Source: CAD feature listing. Evaluate the final solid. Frame: model axes, mm. A direction names the side the tool comes from. Give positions to 0.01 mm unless a question says otherwise; leave off trailing zeros. Loops run counter-clockwise (first coordinate to the right, second up) from the corner with the lowest first, then second, coordinate; pieces in that order, holes last. Notation, with made-up numbers: M 79.5,64.25 L 131.5,64.25 A18 ccw 131.5,71.25 Z; hole C 15,36 d7. An arc over 180 degrees is marked long. Put each result on its own line as item: value.
from build123d import *

# Parameters (mm, degrees)
SKETCH_1_W          = 50
SKETCH_1_H          = 20
EXTRUDE_1_DEPTH     = 180
CUT_EXTRUDE_1_DEPTH = 10
CUT_EXTRUDE_2_DEPTH = 10
SKETCH_4_OUTSIDE_W  = 219.576
SKETCH_4_OUTSIDE_H  = 89.576
CUT_EXTRUDE_4_DEPTH = 21


with BuildPart() as part:
    # Эскиз1 → Бобышка-Вытянуть1 (new body)
    with BuildSketch(Plane(origin=(0, 0, 0), x_dir=(0, 0, -1), z_dir=(1, 0, 0))):
        with Locations((25, 10)):
            Rectangle(SKETCH_1_W, SKETCH_1_H)
    extrude(amount=EXTRUDE_1_DEPTH)

    # Эскиз2 → Вырез-Вытянуть1 (cut)
    with BuildSketch(Plane.XZ):
        with BuildLine():
            Line((43.517527849, -50), (0, -50))
            Line((0, -50), (0, 0))
            Line((0, 0), (50.69898236, 0))
            Line((50.69898236, 0), (60.088568146, -16.308535178))
            ThreePointArc((60.088568146, -16.308535178), (60.755434633, -18.806330829), (60.085562557, -21.303322104))
            Line((60.085562557, -21.303322104), (43.517527849, -50))
        make_face()
    extrude(amount=-CUT_EXTRUDE_1_DEPTH, mode=Mode.SUBTRACT)

    # Эскиз3 → Вырез-Вытянуть2 (cut)
    with BuildSketch(Plane(origin=(0, 20, 0), x_dir=(1, 0, 0), z_dir=(0, 1, 0))):
        with BuildLine():
            Line((119.870060572, 21.260602823), (136.462759268, 50))
            Line((136.462759268, 50), (180, 50))
            Line((180, 50), (180, 0))
            Line((180, 0), (129.384239064, 0))
            Line((129.384239064, 0), (119.884637949, 16.23552237))
            ThreePointArc((119.884637949, 16.23552237), (119.200208629, 18.746098263), (119.870060572, 21.260602823))
        make_face()
    extrude(amount=-CUT_EXTRUDE_2_DEPTH, mode=Mode.SUBTRACT)

    # Эскиз4 outside → Вырез-Вытянуть4 (cut, through all)
    with BuildSketch(Plane(origin=(0, 20, 0), x_dir=(1, 0, 0), z_dir=(0, 1, 0))):
        with Locations((90, 25)):
            Rectangle(SKETCH_4_OUTSIDE_W, SKETCH_4_OUTSIDE_H)
        with BuildLine():
            Line((180, 50), (152.575862213, 2.5))
            ThreePointArc((152.575862213, 2.5), (150.745735195, 0.669872981), (148.245735195, 0))
            Line((148.245735195, 0), (31.754264805, 0))
            ThreePointArc((31.754264805, 0), (29.254264805, 0.669872981), (27.424137787, 2.5))
            Line((27.424137787, 2.5), (0, 50))
            Line((0, 50), (180, 50))
        make_face(mode=Mode.SUBTRACT)
    extrude(amount=-CUT_EXTRUDE_4_DEPTH, mode=Mode.SUBTRACT)


solid = part.part
1. Contact query for flat-ended pins moving along their axis: P1, Ø1.5, axis at y = 17.5, z = -12.5, coming from the +X side; P2, Ø5, axis at x = 147, z = -34, coming from the +Y side; P3, Ø10, axis at y = 10.5, z = -21.5, coming from the -X side. Output: stop coordinate, or through.
Found:
P1: x = 122.51
P2: y = 10
P3: x = 13.57
2. Draft query along Z for faces 1 (the flat face through (89, 10, -50)), 2 (the flat face through (111, 0, -25)), 3 (the cylindrical face through (119.2, 15.1, -18.7)), 4 (the flat face through (89, 10, 0)). Return one class per face: pulls with the +Z half, pulls with the -Z half, needs draft (parallel to the pull), parting line crosses it, or undercut.
Found:
face 1: pulls with the -Z half
face 2: needs draft
face 3: undercut
face 4: pulls with the +Z half
3. Material intervals for line 1 (Y direction, x = 29.5, z = -24.5); line 2 (Y direction, x = 150.5, z = -40.5); line 3 (X direction, y = 3, z = -12), sorted ascending. Write a range as from..to.
Found:
line 1: 10..20
line 2: 0..10
line 3: 57.61..158.06
4. Section query C-C (y = 4). Output: boundary loops of the cut face in (x, z), plus the area to 3 significant figures.
Found:
outline: M 43.52,-50 L 180,-50 L 152.58,-2.5 A5 ccw 148.25,0 L 50.7,0 L 60.09,-16.31 A5 cw 60.09,-21.3 Z
area: 5,580 mm^2
5. Section query D-D (x = 157.5). Output: boundary loops of the cut face in (y, z).
Found:
outline: M 0,-50 L 10,-50 L 10,-11.03 L 0,-11.03 Z
6. Access query for faces 5 (the flat face through (13.904, 15.07, -25.918)), 6 (the flat face through (38, 10, -25)), 7 (the flat face through (124.701, 15.07, -8.004)). Directions: +Z, -Z, +X, -X, +Y, -Y. A direction counts if a zero-diameter tool reaches every point of the face in a straight line with its end or side. Return the directions, or none.
Found:
face 5: +Z, -X, +Y, -Y
face 6: -X, -Y
face 7: +X, +Y
7. Section query A-A (y = 13). Output: boundary loops of the cut face in (x, z).
Found:
outline: M 0,-50 L 136.46,-50 L 119.87,-21.26 A5 cw 119.88,-16.24 L 129.38,0 L 31.75,0 A5 ccw 27.42,-2.5 Z
8. Section query B-B (z = -31.5). Output: boundary loops of the cut face in (x, y).
Found:
outline: M 10.68,10 L 54.2,10 L 54.2,0 L 169.32,0 L 169.32,10 L 125.78,10 L 125.78,20 L 10.68,20 Z
